Can you work these out from the model? Positions are in its coordinate system, mm. Face numbers are marked on the shaded views. Coordinates: 2 decimals unless noted, no trailing zeros. Order: outer loops, then holes, each group sorted by start corner. A loop starts at its lowest first (then second) coordinate and runs counter-clockwise, first axis right, second up. Notation, with made-up numbers: (2.5, -19) -> (57.5, -19) arc R24 ccw to (57.5, 16) -> close; hole circle Ø6 at (18, 68.5). An arc over 180 degrees is marked (long way). Return JSON: item names as keys, results as strings. Group by question number.
1) If I drill on probe 1 along Y at (x, z) = (0, 8); probe 2 along X at (y, z) = (2.5, 10); probe 3 along X at (y, z) = (-16, 9), over which ranges is the centre line in solid material (lowest first)? Write a range as from..to.
2) If we section it at A-A, the plane y = 0: Please give me the cut outline in (x, z).
3) For pin 1 (8 mm diameter, centred on x = -7.5, z = 15, fed in from -Y); pin 2 (5 mm diameter, centred on x = -9, z = 13, fed in from -Y); pin 3 (12 mm diameter, centred on x = 11.5, z = 16, fed in from -Y), each with a flat end and sliding along its axis, tell me the tip position at first contact or that it passes through.
4) If we section it at C-C, the plane z = 2.5: Please give me the cut outline in (x, y).
5) Thinking about a two-plate mould opening in Y: for the marked faces 1, 2 and 3, which applies, +Y half, -Y half, draft (parallel to the pull), parting line (faces both ways), or undercut?
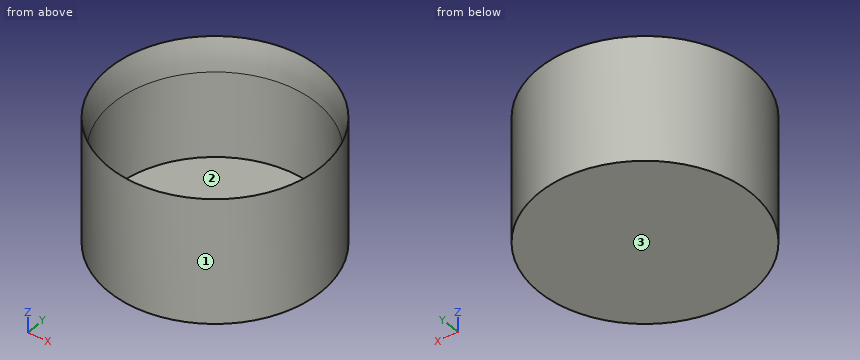
from build123d import *

# Parameters (mm, degrees)
F0_R     = 18.923
F0_R_2   = 18.161
F1_DEPTH = 22.352
F2_R     = 18.8764388906
F3_DEPTH = 1.27


# Not quite as in the source:
# - a fillet or chamfer that OpenCascade refuses, or shapes differently, is made with other operations: its cross-section is extruded or revolved along the edge and cut away or added


with BuildPart() as f1:
    # F0 (on Top) → F1 (new body)
    with BuildSketch(Plane.XY):
        Circle(F0_R)
        Circle(F0_R_2, mode=Mode.SUBTRACT)
    extrude(amount=F1_DEPTH)

    # F2 (on Top) → F3 (join)
    with BuildSketch(Plane.XY):
        Circle(F2_R)
    extrude(amount=F3_DEPTH)

    # F4: fillet of radius 22.86 on 1 edges, made by hand

    # F4_s1 → F4_t2 (revolve, cut)
    with BuildSketch(Plane.XZ):
        with BuildLine():
            ThreePointArc((18.923, 22.352), (18.3523004343, 19.4501802499), (18.161, 16.4989669401))
            Line((18.161, 16.4989669401), (18.161, 22.352))
            Line((18.161, 22.352), (18.923, 22.352))
        make_face()
    revolve(axis=Axis((0, 0, 22.352), (0, 0, 1)), mode=Mode.SUBTRACT)


solid = f1.part
Result sheet:
{
 "1": {"probe 1": "y = -18.92..-18.16, 18.16..18.92", "probe 2": "x = -18.76..-17.99, 17.99..18.76", "probe 3": "x = -10.1..-8.59, 8.59..10.1"},
 "2": {"outline": "(-18.92, 0) -> (18.92, 0) -> (18.92, 22.35) arc R22.86 ccw to (18.16, 16.5) -> (18.16, 1.27) -> (-18.16, 1.27) -> (-18.16, 16.5) arc R22.86 ccw to (-18.92, 22.35) -> close"},
 "3": {"pin 1": "stops at y = -18.6", "pin 2": "stops at y = -17.77", "pin 3": "stops at y = -18.11"},
 "4": {"outline": "circle Ø37.85 at (0, 0); hole circle Ø36.32 at (0, 0)"},
 "5": {"face 1": "parting line", "face 2": "undercut", "face 3": "draft"}
}
